The listing builds one solid part. Answer for the finished solid, in the listing's coordinates (mm). Face numbers are marked on the shaded views. Give positions to 0.01 mm unless a question says otherwise; leave off trailing zeros. Order: outer loops, then holes, each group sorted by start corner. A loop starts at its lowest first (then second) coordinate and runs counter-clockwise, first axis right, second up. Notation, with made-up numbers: (61.5, 77) - (75.5, 77) arc R16 ccw to (75.5, 86) - close; hole circle Ø5 at (12.5, 78). An arc over 180 degrees is marked (long way). Answer as a JSON object with one key per item and string values. Group by question number.
Q1. A cutting plane is placed at C-C, the plane y = 14. Give the vertices of the cut face in (x, z), and give its area (3 significant figures).
Q2. A cutting plane is placed at B-B, the plane z = 0.9. Give the vertices of the cut face in (x, y), and give its area (3 significant figures).
Q3. The mould has two halves that part along X. Classify the marked faces 1 and 2: released by +X, released by -X, zero draft, split by the parting line, or undercut.
Q4. A cutting plane is placed at D-D, the plane x = -46. Give the vertices of the cut face in (y, z).
Q5. A cutting plane is placed at A-A, the plane z = 4.55. Give the vertices of the cut face in (x, y) (3 decimals), and give its area (3 significant figures).
Q6. Consider line 1 (Y direction, x = -14.25, z = 3.1) (3 decimals); line 2 (X direction, y = 4.5, z = 2.15); line 3 (X direction, y = 25.75, z = 4.2). Determine where each line is inside the solid, lowest interval first.
Q7. Given pin 1 (7 mm diameter, centred on x = -5, y = 15, fed in from +Z), flat-ended and moving along its own axis, determine where the tip first touches the part or whether it passes through.
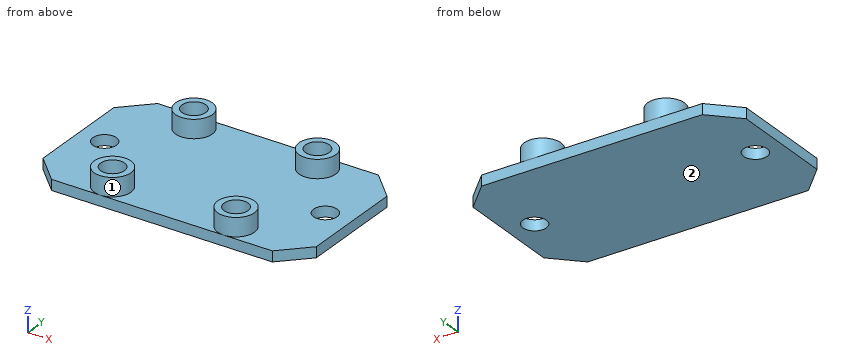
from build123d import *

# Parameters (mm, degrees)
SKETCH_1_W          = 30
SKETCH_1_H          = 52
EXTRUDE_1_DEPTH     = 2
SKETCH_2_R          = 3.5
EXTRUDE_2_DEPTH     = 3.5
SKETCH_5_R          = 2.275
CUT_EXTRUDE_1_DEPTH = 3.5
HOLE_WIZARD_M4_1_D  = 4.5
CHAMFER_1_SIZE      = 5


with BuildPart() as part:
    # ｽｹｯﾁ1 → ﾎﾞｽ - 押し出し1 (new body)
    with BuildSketch(Plane(origin=(0, 0, 0), x_dir=(0, 1, 0), z_dir=(0, 0, 1))):
        with Locations((15, 26)):
            Rectangle(SKETCH_1_W, SKETCH_1_H)
    extrude(amount=EXTRUDE_1_DEPTH)

    # ｽｹｯﾁ2 → ﾎﾞｽ - 押し出し2 (add)
    with BuildSketch(Plane.XY.offset(2)):
        with Locations((-37.75, 26.5)):
            Circle(SKETCH_2_R)
        with Locations((-14.25, 26.5)):
            Circle(SKETCH_2_R)
        with Locations((-14.25, 3.5)):
            Circle(SKETCH_2_R)
        with Locations((-37.75, 3.5)):
            Circle(SKETCH_2_R)
    extrude(amount=EXTRUDE_2_DEPTH)

    # ｽｹｯﾁ5 → ｶｯﾄ - 押し出し1 (cut)
    with BuildSketch(Plane.XY.offset(5.5)):
        with Locations((-37.75, 26.5)):
            Circle(SKETCH_5_R)
        with Locations((-14.25, 26.5)):
            Circle(SKETCH_5_R)
        with Locations((-14.25, 3.5)):
            Circle(SKETCH_5_R)
        with Locations((-37.75, 3.5)):
            Circle(SKETCH_5_R)
    extrude(amount=-CUT_EXTRUDE_1_DEPTH, mode=Mode.SUBTRACT)

    # M4 すきま穴1 (through all)
    with Locations(Plane.XY.offset(2)):
        with Locations((-47, 15), (-5, 15)):
            Hole(HOLE_WIZARD_M4_1_D / 2)

    # 面取り1
    chamfer_1_edges = [part.edges().sort_by_distance(p)[0] for p in [
        (-52, 0, 1),
        (-52, 30, 1),
        (0, 30, 1),
        (0, 0, 1),
    ]]
    chamfer(chamfer_1_edges, length=CHAMFER_1_SIZE)


solid = part.part
Reply:
{
 "1": {"outline": "(-52, 0) - (-49.02, 0) - (-49.02, 2) - (-52, 2) - close; (-44.98, 0) - (-7.02, 0) - (-7.02, 2) - (-44.98, 2) - close; (-2.98, 0) - (0, 0) - (0, 2) - (-2.98, 2) - close", "area": "87.9 mm^2"},
 "2": {"outline": "(-52, 5) - (-47, 0) - (-5, 0) - (0, 5) - (0, 25) - (-5, 30) - (-47, 30) - (-52, 25) - close; hole circle Ø4.5 at (-47, 15); hole circle Ø4.5 at (-5, 15)", "area": "1,480 mm^2"},
 "3": {"face 1": "undercut", "face 2": "zero draft"},
 "4": {"outline": "(0, 0) - (12.98, 0) - (12.98, 2) - (0, 2) - close; (17.02, 0) - (30, 0) - (30, 2) - (17.02, 2) - close"},
 "5": {"outline": "circle Ø7 at (-37.75, 3.5); circle Ø7 at (-37.75, 26.5); circle Ø7 at (-14.25, 3.5); circle Ø7 at (-14.25, 26.5); hole circle Ø4.55 at (-37.75, 3.5); hole circle Ø4.55 at (-37.75, 26.5); hole circle Ø4.55 at (-14.25, 3.5); hole circle Ø4.55 at (-14.25, 26.5)", "area": "88.9 mm^2"},
 "6": {"line 1": "y = 0 to 1.225, 5.775 to 7, 23 to 24.225, 28.775 to 30", "line 2": "x = -41.1 to -39.79, -35.71 to -34.4, -17.6 to -16.29, -12.21 to -10.9", "line 3": "x = -41.17 to -39.9, -35.6 to -34.33, -17.67 to -16.4, -12.1 to -10.83"},
 "7": {"pin 1": "stops at z = 2"}
}
